```python
from build123d import *

# Parameters (mm, degrees)
F1_DEPTH = 7.25
F3_DEPTH = 2.25
F3_TAPER = 45
F4_DEPTH = 2.25
F4_TAPER = 45
F5_DEPTH = 5


with BuildPart() as f1:
    # F0 (on Front) → F1 (new body)
    with BuildSketch(Plane.XZ):
        with BuildLine():
            Line((-45, 0), (-30, 0))
            Line((-30, 0), (-30, 5))
            ThreePointArc((-30, 5), (-15, 19), (0, 5))
            Line((0, 5), (0, 0))
            Line((0, 0), (15, 0))
            Line((15, 0), (15, 7.25))
            ThreePointArc((15, 7.25), (-15, 39), (-45, 7.25))
            Line((-45, 7.25), (-45, 0))
        make_face()
    extrude(amount=F1_DEPTH)

    # F2 (on face) → F3 (join)
    with BuildSketch(Plane.XZ.offset(7.25)):
        with BuildLine():
            ThreePointArc((15, 7.25), (-15, 39), (-45, 7.25))
            Line((-45, 7.25), (-45, 0))
            Line((-45, 0), (-30, 0))
            Line((-30, 0), (-30, 5))
            ThreePointArc((-30, 5), (-15, 19), (0, 5))
            Line((0, 5), (0, 0))
            Line((0, 0), (15, 0))
            Line((15, 0), (15, 7.25))
        make_face()
    extrude(amount=F3_DEPTH, taper=F3_TAPER)

    # F1_face1 (on face) → F4 (join)
    with BuildSketch(Plane(origin=(-15, 0, 19.7628829263), x_dir=(1, 0, 0), z_dir=(0, 1, 0))):
        with BuildLine():
            Line((-30, 19.7628829263), (-30, 12.5128829263))
            ThreePointArc((-30, 12.5128829263), (0, -19.2371170737), (30, 12.5128829263))
            Line((30, 12.5128829263), (30, 19.7628829263))
            Line((30, 19.7628829263), (15, 19.7628829263))
            Line((15, 19.7628829263), (15, 14.7628829263))
            ThreePointArc((15, 14.7628829263), (0, 0.7628829263), (-15, 14.7628829263))
            Line((-15, 14.7628829263), (-15, 19.7628829263))
            Line((-15, 19.7628829263), (-30, 19.7628829263))
        make_face()
    extrude(amount=F4_DEPTH, taper=F4_TAPER)

    # F5 (add): a face of the model
    f5_faces = [f1.faces().sort_by_distance(p)[0] for p in [
        (7.5, -3.625, 0),
    ]]
    extrude(f5_faces, amount=F5_DEPTH)


solid = f1.part
```
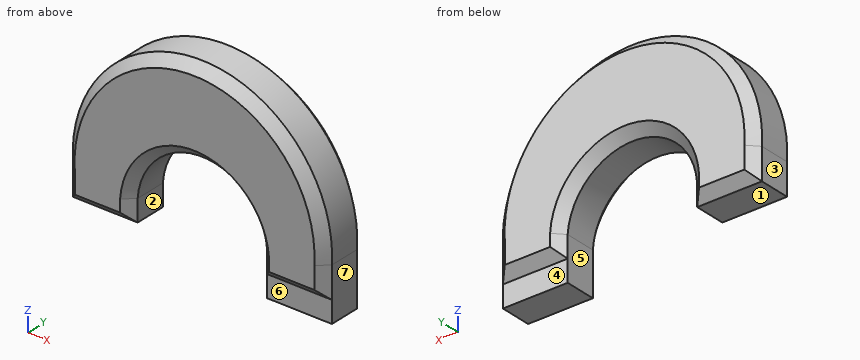
Model file for the job. Use its own axes, mm. Face numbers are marked on the shaded views. A direction names the side the tool comes from. Coordinates: 2 decimals unless noted, no trailing zeros. Write each loop counter-clockwise with the first axis right and the second up, starting at its lowest first coordinate (ties: lowest second). Pieces come first, ordered by that corner, then holes. Notation, with made-up numbers: (-18.5, 5.25) - (-5.5, 5.25) arc R33 ccw to (-5.5, 39.25) - close; hole circle Ø1 at (19.5, 14). An arc over 180 degrees is marked (long way). Use a Markdown table: item, result. Add a question column.
Item 1: Two-plate mould, pull along X, no slides. Class the marked faces 1, 2 and 3: pulls with the +X half, pulls with the -X half, needs draft (parallel to the pull), parting line crosses it, or undercut.
Item 2: Drop flat-ended pins along their axis: pin 1 (4 mm diameter, centred on x = 8.5, z = -2.5, fed in from +Y); pin 2 (6 mm diameter, centred on y = -8, z = 17.5, fed in from +X); pin 3 (4 mm diameter, centred on y = -4, z = 2, fed in from +X). Give the stop position or say it passes through.
Item 3: Band-saw the part on A-A, the plane y = -5.5. Write the cut outline in (x, z).
Item 4: 3-axis set-ups, long thin cutter, end or side, ignore diameter. For the marked faces 4, 5, 6 and 7: which of +Z, -Z, +X, -X, +Y, -Y reach the whole face in a straight line?
Item 5: Drill centre lines: line 1 along X through (y, z) = (-4, 2.5); line 2 along X through (y, z) = (0, 10); line 3 along X through (y, z) = (1.25, 33). Where is each one in solid material? Low to high.
A:
| question | item | result |
|---|---|---|
| 1 | face 1 | needs draft |
| 1 | face 2 | undercut |
| 1 | face 3 | pulls with the -X half |
| 2 | pin 1 | stops at y = 0 |
| 2 | pin 2 | stops at x = 14.51 |
| 2 | pin 3 | stops at x = 15 |
| 3 | outline | (-45, 0) - (-30, 0) - (-30, 5) arc R15.04 cw to (0, 5) - (0, -5) - (15, -5) - (15, 7.25) arc R30.05 ccw (long way) to (-45, 7.25) - close |
| 4 | face 4 | -Z, +X, -X, +Y |
| 4 | face 5 | -Z, +Y, -Y |
| 4 | face 6 | -Z, +X, -X, -Y |
| 4 | face 7 | -Z, +X, +Y, -Y |
| 5 | line 1 | x = -45 to -30, 0 to 15 |
| 5 | line 2 | x = -45.03 to -28.77, -1.23 to 15.03 |
| 5 | line 3 | x = -30.84 to 0.84 |
